```python
from build123d import *

# Parameters (mm, degrees)
BOSS_EXTRUDE1_DEPTH                = 5
BASE_SKETCH_4_W                    = 4.5
BASE_SKETCH_4_H                    = 2.75
BOSS_EXTRUDE2_DEPTH                = 5
TAP_DRILL_FOR_M1_2X0_25_TAP1_D     = 0.95
TAP_DRILL_FOR_M1_2X0_25_TAP1_DEPTH = 1.739637029


with BuildPart() as part:
    # base_sketch<3> → Boss-Extrude1 (new body)
    with BuildSketch(Plane(origin=(0, 0, 0), x_dir=(0, 0, -1), z_dir=(1, 0, 0))):
        Polygon((-1.75, -1.010362971), (-1.166666667, 0), (-2.25, 0), (-2.25, -2.75), (2.25, -2.75), (2.25, 0), (1.166666667, 0), (1.75, -1.010362971), align=None)
    extrude(amount=BOSS_EXTRUDE1_DEPTH)

    # base_sketch<4> → Boss-Extrude2 (add)
    with BuildSketch(Plane(origin=(0, 0, 0), x_dir=(0, 0, -1), z_dir=(1, 0, 0))):
        with Locations((0, -1.375)):
            Rectangle(BASE_SKETCH_4_W, BASE_SKETCH_4_H)
    extrude(amount=-BOSS_EXTRUDE2_DEPTH)

    # Tap Drill for M1.2x0.25 Tap1
    with Locations(Plane(origin=(0, -2.75, 0), x_dir=(-1, 0, 0), z_dir=(0, -1, 0))):
        with Locations((-4, 0), (-2, 0)):
            Hole(TAP_DRILL_FOR_M1_2X0_25_TAP1_D / 2, depth=TAP_DRILL_FOR_M1_2X0_25_TAP1_DEPTH)


solid = part.part
```
Model file for the job. Use its own axes, mm. A direction names the side the tool comes from. Give positions to 0.01 mm unless a question says otherwise; leave off trailing zeros. Order: outer loops, then holes, each group sorted by start corner. A loop starts at its lowest first (then second) coordinate and runs counter-clockwise, first axis right, second up.
1) Mould opens along Z. For faces 1 (the flat face through (2.5, -1.01, -0.4)), 2 (the flat face through (0, -1, -2.25)), 3 (the flat face through (-5, -1, 0)), 4 (the cylindrical face through (1.525, -1.868, -0.021)) say: +Z half, -Z half, draft (parallel to the pull), parting line (faces both ways), or undercut.
2) Pin check, flat tip, straight feed: pin 1 (0.5 mm diameter, centred on y = -0.5, z = 0, fed in from +X). Stop position of the tip, or through.
3) Saw through at D-D, the plane y = -1.25. Write the cut outline in (x, z) (3 decimals), then the cut area to 3 significant figures.
4) Saw through at B-B, the plane z = -0.15. Write the cut outline in (x, y), then the cut area to 3 significant figures.
5) Saw through at A-A, the plane x = 4. Write the cut outline in (y, z) (3 decimals).
6) 3-axis set-ups, long thin cutter, end or side, ignore diameter. For faces 5 (the flat face through (0, -1, 2.25)), 6 (the flat face through (2.46, -0.51, 1.46)): which of +Z, -Z, +X, -X, +Y, -Y reach the whole face in a straight line?
7) Wall check: probe 1 along Z at (x, y) = (2, -2) (3 decimals); probe 2 along Y at (x, z) = (1.75, 1.1); probe 3 along Y at (x, z) = (1.5, -1.65). Give the ranges that are in metal, low to high.
8) Saw through at C-C, the plane x = 0.5. Write the cut outline in (y, z).
Computed:
1. face 1: undercut
1. face 2: -Z half
1. face 3: draft
1. face 4: undercut
2. pin 1: stops at x = 0
3. outline: (-5, -2.25) - (5, -2.25) - (5, 2.25) - (-5, 2.25) - close; hole circle Ø0.95 at (2, 0); hole circle Ø0.95 at (4, 0)
3. area: 43.6 mm2
4. outline: (-5, -2.75) - (1.55, -2.75) - (1.55, -1.01) - (0, -1.01) - (0, 0) - (-5, 0) - close; (2.45, -2.75) - (3.55, -2.75) - (3.55, -1.01) - (2.45, -1.01) - close; (4.45, -2.75) - (5, -2.75) - (5, -1.01) - (4.45, -1.01) - close
4. area: 19.3 mm2
5. outline: (-2.75, -2.25) - (0, -2.25) - (0, -1.167) - (-1.01, -1.75) - (-1.01, -0.475) - (-2.75, -0.475) - close; (-2.75, 0.475) - (-1.01, 0.475) - (-1.01, 1.75) - (0, 1.167) - (0, 2.25) - (-2.75, 2.25) - close
6. face 5: +Z, +X, -X, +Y, -Y
6. face 6: +X
7. probe 1: z = -2.25 to -0.475, 0.475 to 2.25
7. probe 2: y = -2.75 to -1.01
7. probe 3: y = -2.75 to -1.01, -0.84 to 0
8. outline: (-2.75, -2.25) - (0, -2.25) - (0, -1.17) - (-1.01, -1.75) - (-1.01, 1.75) - (0, 1.17) - (0, 2.25) - (-2.75, 2.25) - close
